```python
from build123d import *

# Parameters (mm, degrees)
F0_W     = 1
F0_H     = 10
F1_DEPTH = 1.5
F2_DEPTH = 9


with BuildPart() as f1:
    # F0 (on Top) → F1 (new body)
    with BuildSketch(Plane.XY):
        Polygon((-17.5, 26.75), (0, 26.75), (17.5, 26.75), (17.5, 27.75), (0, 27.75), (-17.5, 27.75), align=None)
        Polygon((-17.5, 0), (-17.5, 26.75), (-17.5, 27.75), (-18.5, 27.75), (-18.5, -27.75), (-17.5, -27.75), (-17.5, -26.75), align=None)
        Polygon((17.5, 26.75), (0, 26.75), (-17.5, 26.75), (-17.5, 0), (-17.5, -26.75), (0, -26.75), (17.5, -26.75), (17.5, -16.75), (17.5, -6.75), (17.5, 0), align=None)
        Polygon((0, -26.75), (-17.5, -26.75), (-17.5, -27.75), (0, -27.75), (17.5, -27.75), (17.5, -26.75), align=None)
        Polygon((17.5, 27.75), (17.5, 26.75), (17.5, 0), (17.5, -6.75), (18.5, -6.75), (18.5, 27.75), align=None)
        Polygon((18.5, -16.75), (17.5, -16.75), (17.5, -26.75), (17.5, -27.75), (18.5, -27.75), align=None)
        with Locations((18, -11.75)):
            Rectangle(F0_W, F0_H)
    extrude(amount=F1_DEPTH)

    # F0 (on Top) → F2 (join)
    with BuildSketch(Plane.XY):
        Polygon((-17.5, 0), (-17.5, 26.75), (-17.5, 27.75), (-18.5, 27.75), (-18.5, -27.75), (-17.5, -27.75), (-17.5, -26.75), align=None)
        Polygon((17.5, 27.75), (17.5, 26.75), (17.5, 0), (17.5, -6.75), (18.5, -6.75), (18.5, 27.75), align=None)
        Polygon((18.5, -16.75), (17.5, -16.75), (17.5, -26.75), (17.5, -27.75), (18.5, -27.75), align=None)
    extrude(amount=-F2_DEPTH)


solid = f1.part
```
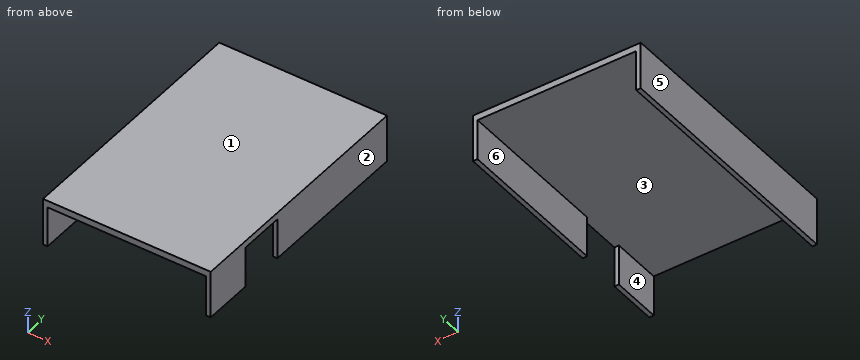
Check sheet for the modelled part. Datum: model origin and axes. Units: mm. Face numbers are marked on the shaded views. A direction names the side the tool comes from. Round coordinates to 2 decimals unless told otherwise and drop trailing zeros. Order: outer loops, then holes, each group sorted by start corner. A loop starts at its lowest first (then second) coordinate and runs counter-clockwise, first axis right, second up.
1) Go/stop test with flat-tipped pins: pin 1 Ø4.5 at (y, z) = (-13, -6) entering from +X; pin 2 Ø1 at (x, z) = (-10, -1.5) entering from -Y; pin 3 Ø12 at (x, y) = (-3, -18.5) entering from -Z. Record where each tip stops, or that it passes through.
2) Section check A-A (z = -4). Record the boundary of the cut face in (x, y), and give its area (3 significant figures).
3) Section check C-C (x = -4.5). Record the boundary of the cut face in (y, z), and give its area (4 significant figures).
4) Section check D-D (y = -11). Record the boundary of the cut face in (x, z), and give its area (3 significant figures).
5) Scan lines: line 1 (X direction, y = 10.5, z = -7.75); line 2 (Z direction, x = 10.5, y = -3); line 3 (X direction, y = -8, z = -5). Record each from-to range of solid material in increasing order.
6) Tool access check on the marked faces 5 and 6. Record the directions out of +Z, -Z, +X, -X, +Y, -Y that give a thin tool (end or side, any length) a straight path to the whole face; none if there is none.
7) Section check B-B (y = -3). Record the boundary of the cut face in (x, z), and give its area (3 significant figures).
8) Mould release check, pull along X, two halves, no side actions. Record for the marked faces 1, 2, 3 and 4: +X half, -X half, draft (parallel to the pull), parting line (faces both ways), or undercut.
Result:
1. pin 1: stops at x = -17.5
1. pin 2: passes through
1. pin 3: stops at z = 0
2. outline: (-18.5, -27.75) - (-17.5, -27.75) - (-17.5, 27.75) - (-18.5, 27.75) - close; (17.5, -27.75) - (18.5, -27.75) - (18.5, -16.75) - (17.5, -16.75) - close; (17.5, -6.75) - (18.5, -6.75) - (18.5, 27.75) - (17.5, 27.75) - close
2. area: 101 mm2
3. outline: (-27.75, 0) - (27.75, 0) - (27.75, 1.5) - (-27.75, 1.5) - close
3. area: 83.25 mm2
4. outline: (-18.5, -9) - (-17.5, -9) - (-17.5, 0) - (18.5, 0) - (18.5, 1.5) - (-18.5, 1.5) - close
4. area: 64.5 mm2
5. line 1: x = -18.5 to -17.5, 17.5 to 18.5
5. line 2: z = 0 to 1.5
5. line 3: x = -18.5 to -17.5
6. face 5: +Z, -Z, -X, +Y, -Y
6. face 6: -Z, +Y, -Y
7. outline: (-18.5, -9) - (-17.5, -9) - (-17.5, 0) - (17.5, 0) - (17.5, -9) - (18.5, -9) - (18.5, 1.5) - (-18.5, 1.5) - close
7. area: 73.5 mm2
8. face 1: draft
8. face 2: +X half
8. face 3: undercut
8. face 4: undercut
